Check sheet for the modelled part. Datum: model origin and axes. Units: mm. Give positions to 0.01 mm unless a question says otherwise; leave off trailing zeros. Order: outer loops, then holes, each group sorted by start corner. A loop starts at its lowest first (then second) coordinate and runs counter-clockwise, first axis right, second up.
Item 1: Sectioned sample at A-A on y = -0.4. Record the boundary of the cut face in (x, z), and give its area (3 significant figures).
Item 2: Material ranges on line 1 along X through (y, z) = (-0.1, -1.5); line 2 along Z through (x, y) = (-0.5, -0.25), recorded low to high.
Item 3: Sectioned sample at B-B on z = -1.4. Record the boundary of the cut face in (x, y).
Item 4: Sectioned sample at C-C on x = 0.5. Record the boundary of the cut face in (y, z), and give its area (3 significant figures).
Autodesk Inventor part; units mm, degrees
ref_plane "YZ Plane" through (0, 0, 0) normal (1, 0, 0) x (0, 1, 0)
ref_plane "XZ Plane" through (0, 0, 0) normal (0, 1, 0) x (-1, 0, 0)
ref_plane "XY Plane" through (0, 0, 0) normal (0, 0, 1) x (1, 0, 0)
sketch "Sketch1" plane through (0, 0, 0) normal (0, 0, 1) x (1, 0, 0)
  line L0 (-10.6243, -0.0072) -> (4.3757, -0.0072)
  line L1 (4.3757, -0.0072) -> (4.3757, -0.5072)
  line L2 (4.3757, -0.5072) -> (-10.6243, -0.5072)
  line L3 (-10.6243, -0.5072) -> (-10.6243, -0.0072)
  point P0 (0, 0)
  dimension "d0" = 0.5
  dimension "d1" = 15
extrude "Extrusion1" add sketch "Sketch1" along normal blind 10
sketch "Sketch2" plane through (-10.6243, -0.0072, 0) normal (0, 1, 0) x (1, 0, 0)
  line L0 (0, 0) -> (15, 0) construction
  line L1 (7.5, 0) -> (7.5, -10.8529) construction
  line L2 (15, -5.4265) -> (-1.0951, -5.4265) construction
  line L3 (5.5, 2) -> (9.5, 2)
  line L4 (9.5, 2) -> (9.5, 0)
  line L5 (9.5, 0) -> (5.5, 0)
  line L6 (5.5, 0) -> (5.5, 2)
  point P0 (10.6243, 0)
  dimension "d4" = 4
  dimension "d5" = 2
extrude "Extrusion2" add sketch "Sketch2" against normal blind 0.5
sketch "Sketch3" plane through (-10.6243, -0.0072, 10) normal (0, 1, 0) x (1, 0, 0)
  line L0 (0, 10) -> (5.5, 10)
  line L1 (0, 10) -> (0, 0)
  line L2 (15, 0) -> (0, 0)
  line L3 (15, 10) -> (15, 0)
  line L4 (9.5, 10) -> (15, 10)
  line L5 (9.5, 12) -> (9.5, 10)
  line L6 (5.5, 12) -> (9.5, 12)
  line L7 (5.5, 10) -> (5.5, 12)
  line L8 (3.116, 10) -> (3.116, 0)
  line L9 (15, 0) -> (0, 0)
  line L10 (15, 10) -> (9.5, 10)
  line L11 (11.884, 10) -> (11.884, 0)
  line L12 (5.5, 12) -> (9.5, 12) construction
  line L13 (7.5, 12) -> (7.5, 0) construction
  point P0 (10.6243, 10)
extrude "Extrusion3" cut sketch "Sketch3" against normal blind 1 contours L0 L8 L2 L1 | L11 L4 L3 L2
sketch "Sketch4" plane through (-5.1243, -0.0072, -2) normal (0, 1, 0) x (1, 0, 0)
  line L0 (8.8107, -14.8925) -> (-5.1696, -14.8925)
  line L1 (-5.1696, -14.8925) -> (-5.1696, -4.6188)
  line L2 (-5.1696, -4.6188) -> (8.8107, -4.6188)
  line L3 (8.8107, -4.6188) -> (8.8107, -14.8925)
  point P0 (5.1243, -2)
extrude "Extrusion4" cut sketch "Sketch4" against normal blind 1
properties part number "Side wall"
Report:
1. outline: (-7.51, 0) - (-5.12, 0) - (-5.12, -2) - (-1.12, -2) - (-1.12, 0) - (1.26, 0) - (1.26, 2.62) - (-7.51, 2.62) - close
1. area: 31.0 mm2
2. line 1: x = -5.12 to -1.12
2. line 2: z = 0 to 2.62
3. outline: (-5.12, -0.51) - (-1.12, -0.51) - (-1.12, -0.01) - (-5.12, -0.01) - close
4. outline: (-0.51, 0) - (-0.01, 0) - (-0.01, 2.62) - (-0.51, 2.62) - close
4. area: 1.31 mm2
